Drawing for the job (mm, zero at the part's lowest x, y, z). A direction names the side the tool comes from. Coordinates: 2 decimals unless noted, no trailing zeros. Write each loop counter-clockwise with the first axis right and the second up, starting at its lowest first coordinate (ties: lowest second). Pieces come first, ordered by that corner, then holes. Notation, with made-up numbers: (47.25, 29.25) - (91.25, 29.25) arc R29 cw to (91.25, 57.25) - close; hole circle Ø8 at (-35, -39.5). An arc over 180 degrees is marked (long way). Write each question's results on one line, items separated by ' | '.
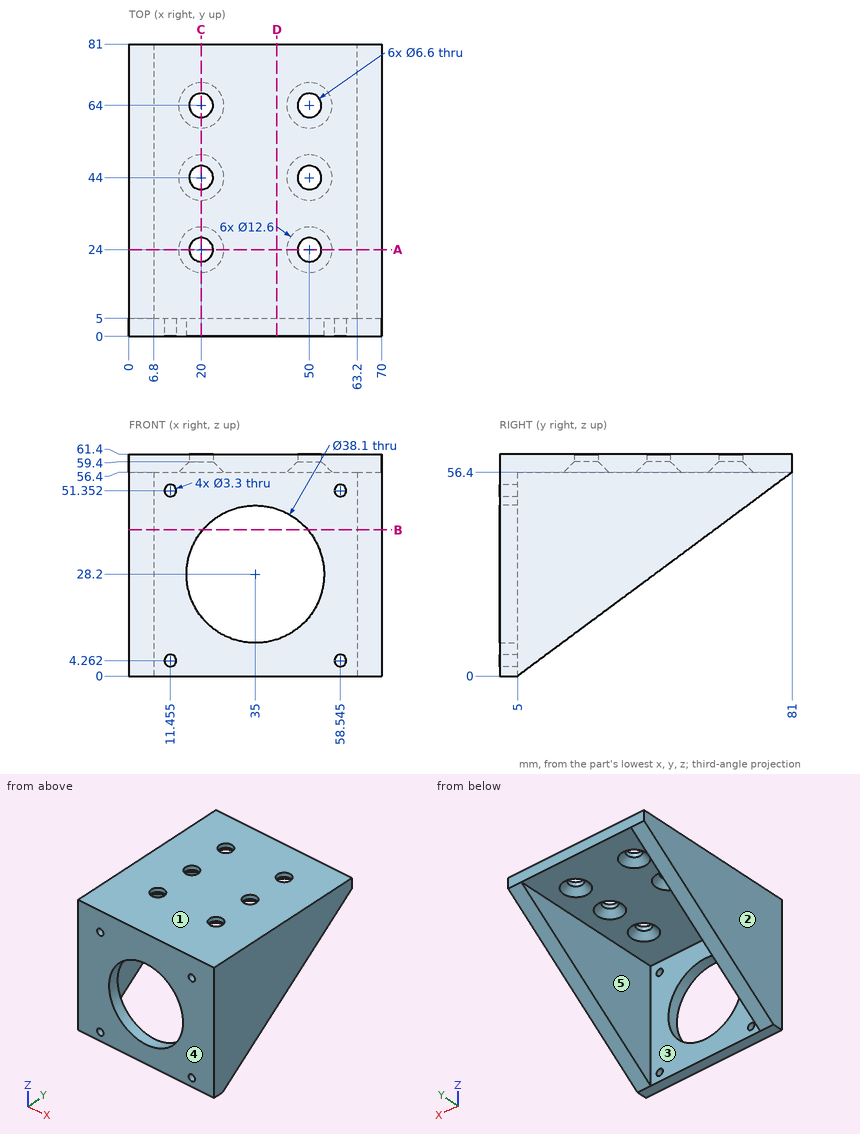
(1) Saw through at B-B on z = 40.5. Write the cut outline in (x, y) (1 decimal).
Return value:
outline: (0, 0) - (20.5, 0) - (20.5, 5) - (6.8, 5) - (6.8, 59.6) - (0, 59.6) - close; (49.5, 0) - (70, 0) - (70, 59.6) - (63.2, 59.6) - (63.2, 5) - (49.5, 5) - close
(2) 3-axis set-ups, long thin cutter, end or side, ignore diameter. For the marked faces 4 and 5: which of +Z, -Z, +X, -X, +Y, -Y reach the whole face in a straight line?
Return value:
face 4: +Z, -Z, +X, -X, -Y | face 5: -Z, +Y
(3) Saw through at A-A on y = 24. Write the cut outline in (x, z).
Return value:
outline: (0, 14.1) - (6.8, 14.1) - (6.8, 56.4) - (13.7, 56.4) - (16.7, 59.4) - (16.7, 61.4) - (0, 61.4) - close; (23.3, 59.4) - (26.3, 56.4) - (43.7, 56.4) - (46.7, 59.4) - (46.7, 61.4) - (23.3, 61.4) - close; (53.3, 59.4) - (56.3, 56.4) - (63.2, 56.4) - (63.2, 14.1) - (70, 14.1) - (70, 61.4) - (53.3, 61.4) - close
(4) Flat gauge pins, fed straight in: P1, Ø3, axis at x = 43, y = 16, coming from the -Z side; P2, Ø4, axis at x = 46.5, z = 47.5, coming from the +Y side; P3, Ø3, axis at x = 58.54, z = 51.35, coming from the +Y side; P4, Ø7.5, axis at x = 20, y = 64, coming from the -Z side. Where does each tip first touch, or does it go through?
Return value:
P1: stops at z = 56.4 | P2: stops at y = 5 | P3: passes through | P4: stops at z = 58.95
(5) Saw through at C-C on x = 20. Write the cut outline in (y, z).
Return value:
outline: (0, 0) - (5, 0) - (5, 16.46) - (0, 16.46) - close; (0, 39.94) - (5, 39.94) - (5, 56.4) - (17.7, 56.4) - (20.7, 59.4) - (20.7, 61.4) - (0, 61.4) - close; (27.3, 59.4) - (30.3, 56.4) - (37.7, 56.4) - (40.7, 59.4) - (40.7, 61.4) - (27.3, 61.4) - close; (47.3, 59.4) - (50.3, 56.4) - (57.7, 56.4) - (60.7, 59.4) - (60.7, 61.4) - (47.3, 61.4) - close; (67.3, 59.4) - (70.3, 56.4) - (81, 56.4) - (81, 61.4) - (67.3, 61.4) - close
(6) Wall check: line 1 (Y direction, x = 50, z = 60); line 2 (X direction, y = 64, z = 60); line 3 (X direction, y = 28, z = 45). Give the ranges that are in metal, low to high. Write a range as from..to.
Return value:
line 1: y = 0..20.7, 27.3..40.7, 47.3..60.7, 67.3..81 | line 2: x = 0..16.7, 23.3..46.7, 53.3..70 | line 3: x = 0..6.8, 63.2..70
(7) Saw through at D-D on x = 41. Write the cut outline in (y, z).
Return value:
outline: (0, 0) - (5, 0) - (5, 10.12) - (0, 10.12) - close; (0, 46.28) - (5, 46.28) - (5, 56.4) - (81, 56.4) - (81, 61.4) - (0, 61.4) - close
(8) Two-plate mould, pull along X, no slides. Class the marked faces 1, 2 and 3: released by +X, released by -X, zero draft, split by the parting line, or undercut.
Return value:
face 1: zero draft | face 2: released by -X | face 3: undercut
